Can you work these out from the model? Positions are in its coordinate system, mm. Round coordinates to 2 decimals unless told otherwise and drop trailing zeros. Write each loop counter-clockwise with the first axis right and the second up, starting at its lowest first coordinate (ties: lowest second). Pieces come first, ordered by that corner, then holes. Notation, with made-up numbers: M -28,-23.75 L 23,-23.75 A32 ccw 23,4.25 Z; hole C -27,-1 d3. An arc over 180 degrees is marked long. Answer as a JSON object with one key per item and string values. Group by question number.
1) I'm going to push flat-ended pins straight in: pin 1 Ø3.5 at (x, z) = (6.5, -1) entering from -Y; pin 2 Ø1.5 at (x, z) = (5.5, -6.5) entering from -Y; pin 3 Ø2 at (x, y) = (5.5, -1.5) entering from +Z. Where does each tip first touch, or does it pass through?
2) Please list where these lines run through material, in increasing order: L1, parallel to Y at x = 9, z = -2; L2, parallel to Y at x = 8.75, z = -6.5; L3, parallel to Z at x = 7, y = -5. Write a range as [from, to].
3) Suppose I cut it at A-A, the plane x = 7.25. Write out the boundary of the cut face in (y, z) (3 decimals), and give its area (3 significant figures).
4) If we mould it in two halves opening along Y, with no side actions, what happens to faces 1 (the flat face through (5, 0, -6)), 2 (the flat face through (5, 0.508, -4))? For each: +Y half, -Y half, draft (parallel to the pull), parting line (faces both ways), or undercut.
from build123d import *

# Parameters (mm, degrees)
SKETCH1_W           = 10.16
SKETCH1_H           = 7.62
BOSS_EXTRUDE1_DEPTH = 0.508
SKETCH2_R           = 3.175
BOSS_EXTRUDE2_DEPTH = 15.24
FILLET1_R           = 3.048
FILLET2_R           = 3.048


with BuildPart() as part:
    # Sketch1 → Boss-Extrude1 (new body)
    with BuildSketch(Plane(origin=(0, 0, 0), x_dir=(1, 0, 0), z_dir=(0, 1, 0))):
        with Locations((5.08, 3.81)):
            Rectangle(SKETCH1_W, SKETCH1_H)
    extrude(amount=BOSS_EXTRUDE1_DEPTH)

    # Sketch2 → Boss-Extrude2 (add)
    with BuildSketch(Plane(origin=(12.7, 0, 0), x_dir=(0, 0, -1), z_dir=(1, 0, 0))):
        with Locations((3.81, -3.080568226)):
            Circle(SKETCH2_R)
    extrude(amount=-BOSS_EXTRUDE2_DEPTH)

    # Fillet1
    # the kernel refuses this fillet: 3.048 mm, written as the material it takes off along each edge
    with BuildSketch(Plane(origin=(-2.54, -3.080568226, -3.81), x_dir=(0, 0, -1), z_dir=(0, -1, 0))) as fillet1_piece_1_section:
        with BuildLine():
            CenterArc((3.175 - FILLET1_R, FILLET1_R), FILLET1_R, 270, 90)
            Line((3.175 - FILLET1_R, 0), (3.175, 0))
            Line((3.175, 0), (3.175, FILLET1_R))
        make_face()
    fillet1_piece_1 = revolve(axis=Axis((-2.54, -3.080568226, -3.81), (1, 0, 0)), mode=Mode.PRIVATE)
    fillet1_piece_1 = split(fillet1_piece_1, bisect_by=Plane(origin=(0, -1.050120042, -6.248507941), z_dir=(1, 0, 0)), keep=Keep.TOP, mode=Mode.PRIVATE)
    fillet1_piece_1 = split(fillet1_piece_1, bisect_by=Plane(origin=(0.252364317, 0, -6.248507941), z_dir=(0, -1, 0)), keep=Keep.TOP, mode=Mode.PRIVATE)
    add(fillet1_piece_1, mode=Mode.SUBTRACT)
    with BuildSketch(Plane(origin=(-2.54, -3.080568226, -3.81), x_dir=(0, 0, -1), z_dir=(0, -1, 0))) as fillet1_piece_2_section:
        with BuildLine():
            CenterArc((3.175 - FILLET1_R, FILLET1_R), FILLET1_R, 270, 90)
            Line((3.175 - FILLET1_R, 0), (3.175, 0))
            Line((3.175, 0), (3.175, FILLET1_R))
        make_face()
    fillet1_piece_2 = revolve(axis=Axis((-2.54, -3.080568226, -3.81), (1, 0, 0)), mode=Mode.PRIVATE)
    fillet1_piece_2 = split(fillet1_piece_2, bisect_by=Plane(origin=(0, -3.080568226, -1.694272015), z_dir=(-1, 0, 0)), keep=Keep.TOP, mode=Mode.PRIVATE)
    fillet1_piece_2 = split(fillet1_piece_2, bisect_by=Plane(origin=(-1.845094679, 0, -1.694272015), z_dir=(0, -1, 0)), keep=Keep.TOP, mode=Mode.PRIVATE)
    add(fillet1_piece_2, mode=Mode.SUBTRACT)
    with BuildSketch(Plane(origin=(-2.54, -3.080568226, -3.81), x_dir=(0, 0, -1), z_dir=(0, -1, 0))) as fillet1_piece_3_section:
        with BuildLine():
            CenterArc((3.175 - FILLET1_R, FILLET1_R), FILLET1_R, 270, 90)
            Line((3.175 - FILLET1_R, 0), (3.175, 0))
            Line((3.175, 0), (3.175, FILLET1_R))
        make_face()
    fillet1_piece_3 = revolve(axis=Axis((-2.54, -3.080568226, -3.81), (1, 0, 0)), mode=Mode.PRIVATE)
    fillet1_piece_3 = split(fillet1_piece_3, bisect_by=Plane(origin=(0, 0.062655826, -3.81), z_dir=(-1, 0, 0)), keep=Keep.TOP, mode=Mode.PRIVATE)
    fillet1_piece_3 = split(fillet1_piece_3, bisect_by=Plane(origin=(-1.310113103, 0, -3.81), z_dir=(0, 1, 0)), keep=Keep.TOP, mode=Mode.PRIVATE)
    add(fillet1_piece_3, mode=Mode.SUBTRACT)

    # Fillet2
    # the kernel refuses this fillet: 3.048 mm, written as the material it takes off along each edge
    with BuildSketch(Plane(origin=(12.7, -3.080568226, -3.81), x_dir=(0, 0, -1), z_dir=(0, -1, 0))) as fillet2_piece_1_section:
        with BuildLine():
            CenterArc((3.175 - FILLET2_R, -FILLET2_R), FILLET2_R, 0, 90)
            Line((3.175 - FILLET2_R, 0), (3.175, 0))
            Line((3.175, 0), (3.175, -FILLET2_R))
        make_face()
    fillet2_piece_1 = revolve(axis=Axis((12.7, -3.080568226, -3.81), (1, 0, 0)), mode=Mode.PRIVATE)
    fillet2_piece_1 = split(fillet2_piece_1, bisect_by=Plane(origin=(9.907635683, 0, -6.248507942), z_dir=(0, -1, 0)), keep=Keep.TOP, mode=Mode.PRIVATE)
    fillet2_piece_1 = split(fillet2_piece_1, bisect_by=Plane(origin=(10.16, -1.050120042, -6.248507942), z_dir=(-1, 0, 0)), keep=Keep.TOP, mode=Mode.PRIVATE)
    add(fillet2_piece_1, mode=Mode.SUBTRACT)
    with BuildSketch(Plane(origin=(12.7, -3.080568226, -3.81), x_dir=(0, 0, -1), z_dir=(0, -1, 0))) as fillet2_piece_2_section:
        with BuildLine():
            CenterArc((3.175 - FILLET2_R, -FILLET2_R), FILLET2_R, 0, 90)
            Line((3.175 - FILLET2_R, 0), (3.175, 0))
            Line((3.175, 0), (3.175, -FILLET2_R))
        make_face()
    fillet2_piece_2 = revolve(axis=Axis((12.7, -3.080568226, -3.81), (1, 0, 0)), mode=Mode.PRIVATE)
    fillet2_piece_2 = split(fillet2_piece_2, bisect_by=Plane(origin=(12.005094679, 0, -1.694272014), z_dir=(0, -1, 0)), keep=Keep.TOP, mode=Mode.PRIVATE)
    fillet2_piece_2 = split(fillet2_piece_2, bisect_by=Plane(origin=(10.16, -3.080568226, -1.694272014), z_dir=(1, 0, 0)), keep=Keep.TOP, mode=Mode.PRIVATE)
    add(fillet2_piece_2, mode=Mode.SUBTRACT)
    with BuildSketch(Plane(origin=(12.7, -3.080568226, -3.81), x_dir=(0, 0, -1), z_dir=(0, -1, 0))) as fillet2_piece_3_section:
        with BuildLine():
            CenterArc((3.175 - FILLET2_R, -FILLET2_R), FILLET2_R, 0, 90)
            Line((3.175 - FILLET2_R, 0), (3.175, 0))
            Line((3.175, 0), (3.175, -FILLET2_R))
        make_face()
    fillet2_piece_3 = revolve(axis=Axis((12.7, -3.080568226, -3.81), (1, 0, 0)), mode=Mode.PRIVATE)
    fillet2_piece_3 = split(fillet2_piece_3, bisect_by=Plane(origin=(11.470113103, 0, -3.81), z_dir=(0, 1, 0)), keep=Keep.TOP, mode=Mode.PRIVATE)
    fillet2_piece_3 = split(fillet2_piece_3, bisect_by=Plane(origin=(10.16, 0.062655826, -3.81), z_dir=(1, 0, 0)), keep=Keep.TOP, mode=Mode.PRIVATE)
    add(fillet2_piece_3, mode=Mode.SUBTRACT)


solid = part.part
Results:
{
 "1": {"pin 1": "y = -6.07", "pin 2": "y = -5.59", "pin 3": "z = -0.69"},
 "2": {"L1": "[-5.69, -0.47], [0, 0.51]", "L2": "[-4.77, -1.39], [0, 0.51]", "L3": "[-6.34, -1.28]"},
 "3": {"outline": "M 0,-7.62 L 0.508,-7.62 L 0.508,0 L 0,0 L 0,-3.041 A3.175 ccw long 0,-4.579 Z", "area": "35.4 mm^2"},
 "4": {"face 1": "undercut", "face 2": "+Y half"}
}
